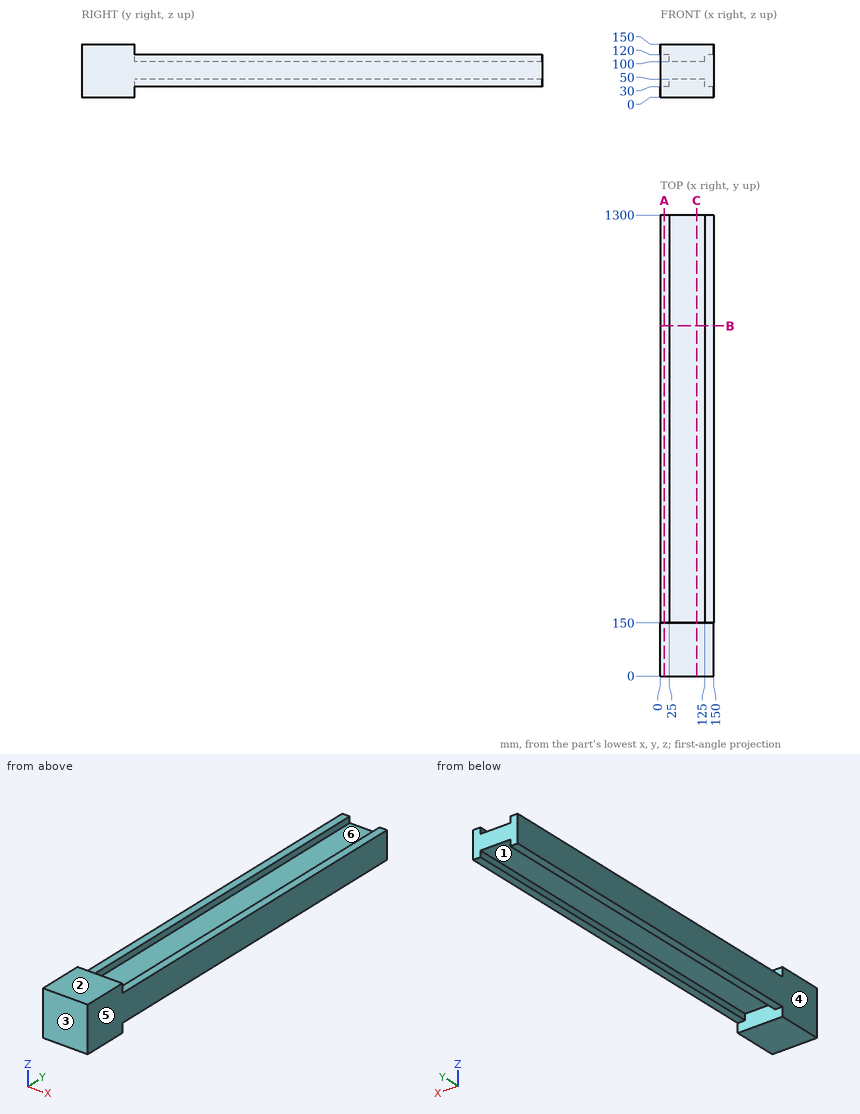
Print and shaded views of the part. All mm, measured from the part's lowest x, y and z. A direction names the side the tool comes from. Round coordinates to 2 decimals unless told otherwise and drop trailing zeros. Write each loop counter-clockwise with the first axis right and the second up, starting at its lowest first coordinate (ties: lowest second). Pieces come first, ordered by that corner, then holes. Notation, with made-up numbers: (24.5, 14.25) - (63.5, 14.25) arc R11 ccw to (63.5, 19.25) - close; hole circle Ø5 at (81.25, 63.5). An arc over 180 degrees is marked (long way). Use CSV: the item, a comma, the result in double quotes. Start each with the question number.
Item 1: Two-plate mould, pull along X, no slides. Class the marked faces 3, 4, 5 and 6: released by +X, released by -X, zero draft, split by the parting line, or undercut.
Item 2: Band-saw the part on C-C (x = 102.5). Write the cut outline in (y, z).
Item 3: Pin check, flat tips, straight feed: P1, Ø10, axis at x = 68, z = 123.5, coming from the +Y side; P2, Ø8, axis at x = 67, y = 541, coming from the +Z side; P3, Ø20, axis at x = 16.5, y = 596.5, coming from the +Z side. Stop position of each tip, or through.
Item 4: Tool access for the marked faces 1 and 2: list every direction of +Z, -Z, +X, -X, +Y, -Y with a clear straight run to the whole face (end or side of a thin tool).
Item 5: Band-saw the part on B-B (y = 987.5). Write the cut outline in (x, z), and give its area (3 significant figures).
Item 6: Band-saw the part on A-A (x = 11.5). Write the cut outline in (y, z), and give its area (3 significant figures).
Item 7: Drill centre lines: L1, parallel to X at y = 790, z = 42; L2, parallel to Y at x = 57.5, z = 36; L3, parallel to Z at x = 70, y = 1105.5. Where is each one in solid material? Low to high. Write a range as [from, to].
Checked values:
1,face 3,"zero draft"
1,face 4,"released by -X"
1,face 5,"released by +X"
1,face 6,"undercut"
2,outline,"(0, 0) - (150, 0) - (150, 50) - (1300, 50) - (1300, 100) - (150, 100) - (150, 150) - (0, 150) - close"
3,P1,"stops at y = 150"
3,P2,"stops at z = 100"
3,P3,"stops at z = 120"
4,face 1,"-Z, +Y"
4,face 2,"+Z, +X, -X, +Y, -Y"
5,outline,"(0, 30) - (25, 30) - (25, 50) - (125, 50) - (125, 30) - (150, 30) - (150, 120) - (125, 120) - (125, 100) - (25, 100) - (25, 120) - (0, 120) - close"
5,area,"9,500 mm²"
6,outline,"(0, 0) - (150, 0) - (150, 30) - (1300, 30) - (1300, 120) - (150, 120) - (150, 150) - (0, 150) - close"
6,area,"126,000 mm²"
7,L1,"x = [0, 25], [125, 150]"
7,L2,"y = [0, 150]"
7,L3,"z = [50, 100]"
